Design review of the part built by this model. Coordinates are the model's own, in mm. A direction names the side the tool comes from. Coordinates: 2 decimals unless noted, no trailing zeros. Write each loop counter-clockwise with the first axis right and the second up, starting at its lowest first coordinate (ties: lowest second). Pieces come first, ordered by that corner, then holes.
Q1. Machinability: for faces 1 (the flat face through (-3.75, 3, 40)), 2 (the cylindrical face through (-32.93, 2.03, 49.4)), 3 (the flat face through (4, 2.5, -3)), 4 (the flat face through (-26, 2, -27)), 5 (the flat face through (20.5, 3, 16)), which of the approach directions +Z, -Z, +X, -X, +Y, -Y give a long, thin tool a straight path to every point of the face, cutting with its end or side? Answer none if there is none.
Q2. Take a section at C-C (x = 16). State how many separate pieces and enclosed holes the cut face has, and give its area (3 significant figures).
Q3. Mouldability with a two-part tool opening along X and no side actions: class faces 6 (the flat face through (29, 3, 35.5)), 7 (the cylindrical face through (32.93, 2.03, -49.4)), 8 (the flat face through (5, 1, -3.5)) as pulls with the +X half, pulls with the -X half, needs draft (parallel to the pull), parting line crosses it, or undercut.
Q4. Take a section at A-A (z = -13). Give the boundary of the cut face in (x, y), and give its area (3 significant figures).
Q5. For probe 1 along Z at (x, y) = (-31, 3.55); probe 2 along X at (y, z) = (0.2, -32); probe 3 along X at (y, z) = (2.2, -6), list the stretches that pass through material, from the lowest coordinate up.
Q6. Take a section at B-B (x = 26). Give the boundary of the cut face in (y, z), and give its area (3 significant figures).
Q7. Insertion check: pin 1 (1 mm diameter, centred on x = -23.5, y = 3, fed in from +Z); pin 2 (0.8 mm diameter, centred on x = -25.5, z = -28, fed in from -Y); pin 3 (3.5 mm diameter, centred on x = -27.5, z = -28.5, fed in from -Y). Each pin has a flat end and moves straight along its axis. Give the tip position at first contact, or say it passes through.
Autodesk Inventor part; units mm, degrees
ref_plane "YZ Plane" through (0, 0, 0) normal (1, 0, 0) x (0, 1, 0)
ref_plane "XZ Plane" through (0, 0, 0) normal (0, 1, 0) x (-1, 0, 0)
ref_plane "XY Plane" through (0, 0, 0) normal (0, 0, 1) x (1, 0, 0)
sketch "Sketch2" plane through (0, 0, 0) normal (0, 1, 0) x (-1, 0, 0)
  line L0 (-33.5, -50) -> (33.5, -50)
  line L1 (33.5, -50) -> (33.5, 50)
  line L2 (33.5, 50) -> (-33.5, 50)
  line L3 (-33.5, 50) -> (-33.5, -50)
  line L4 (-33.5, -50) -> (33.5, 50) construction
  line L5 (33.5, -50) -> (-33.5, 50) construction
  point P0 (0, 0)
  dimension "d0" = 67
  dimension "d1" = 100
extrude "Extrusion1" add sketch "Sketch2" along normal blind 4
sketch "Sketch3" plane through (0, 4, 0) normal (0, 1, 0) x (1, 0, 0)
  line L0 (33.5, 50) -> (-33.5, 50)
  line L1 (-14.5, -6.5) -> (23.5, -6.5)
  line L2 (23.5, -6.5) -> (23.5, 46)
  line L3 (23.5, 46) -> (-14.5, 46)
  line L4 (-14.5, 46) -> (-14.5, -6.5)
  line L5 (-14.5, -6.5) -> (23.5, 46) construction
  line L6 (23.5, -6.5) -> (-14.5, 46) construction
  line L7 (33.5, -50) -> (33.5, 50)
  point P0 (0, 0)
  point P1 (4.5, 19.75)
  dimension "d4" = 38
  dimension "d5" = 52.5
  dimension "d6" = 4
  dimension "d99" = 10
extrude "Extrusion2" cut sketch "Sketch3" against normal blind 1.5
sketch "Sketch4" plane through (0, 2.5, 0) normal (0, 1, 0) x (1, 0, 0)
  line L0 (23.5, -6.5) -> (-14.5, -6.5)
  line L1 (23.5, 46) -> (23.5, -6.5)
  line L2 (-14.5, 46) -> (23.5, 46)
  line L3 (-14.5, -6.5) -> (-14.5, 46)
  line L4 (-12, 44.5) -> (21, 44.5)
  line L5 (21, 44.5) -> (21, 3.5)
  line L6 (21, 3.5) -> (-12, 3.5)
  line L7 (-12, 3.5) -> (-12, 44.5)
  line L8 (-12, 44.5) -> (21, 3.5) construction
  line L9 (21, 44.5) -> (-12, 3.5) construction
  point P0 (0, 0)
  point P1 (4.5, 24)
  dimension "d9" = 10
  dimension "d10" = 1.5
  dimension "d11" = 2.5
  dimension "d12" = 2.5
extrude "Extrusion3" cut sketch "Sketch4" against normal blind 2.5 contours L4 L5 L6 L7
sketch "Sketch5" plane through (0, 4, 0) normal (0, 1, 0) x (1, 0, 0)
  line L0 (23.5, 46) -> (23.5, -6.5)
  line L1 (23.5, -6.5) -> (-14.5, -6.5)
  line L2 (-14.5, -6.5) -> (-14.5, 46)
  line L3 (-12.5, -13) -> (-12.5, -6.5)
  line L4 (21.5, -13) -> (21.5, -6.5)
  line L5 (33.5, 50) -> (-33.5, 50)
  line L6 (-12.5, -13) -> (21.5, -13)
  point P0 (0, 0)
  dimension "d18" = 2
  dimension "d19" = 2
  dimension "d158" = 6.5
extrude "Extrusion4" cut sketch "Sketch5" against normal blind 0.25
sketch "Sketch12" plane through (0, 4, 0) normal (0, 1, 0) x (1, 0, 0)
  line L0 (21.5, -13) -> (-12.5, -13)
  line L1 (-13.5, -37) -> (24.5, -37)
  line L2 (24.5, -37) -> (24.5, -13)
  line L3 (24.5, -13) -> (-13.5, -13)
  line L4 (-13.5, -13) -> (-13.5, -37)
  line L5 (-13.5, -37) -> (24.5, -13) construction
  line L6 (24.5, -37) -> (-13.5, -13) construction
  line L7 (23.5, 46) -> (23.5, -6.5)
  point P0 (0, 0)
  point P1 (5.5, -25)
  point P2 (5.5, -25)
  dimension "d58" = 38
  dimension "d59" = 24
  dimension "d100" = 1
extrude "Extrusion10" cut sketch "Sketch12" against normal blind 4
sketch "Sketch13" plane through (24.5, 4, 13) normal (-1, 0, 0) x (0, 0, 1)
  line L0 (0, 0) -> (24, 0)
  line L1 (0, 0) -> (0, -4)
  line L2 (24, -4) -> (0, -4)
  line L3 (6, 0) -> (6, -4)
  line L4 (0, -2.2) -> (6, -2.2)
  point P0 (-13, -4)
  dimension "d67" = 6
  dimension "d74" = 1.8
sketch "Sketch14" plane through (-13.5, 4, 37) normal (1, 0, 0) x (0, 0, -1)
  line L0 (0, 0) -> (24, 0)
  line L1 (0, 0) -> (0, -4)
  line L2 (4, -2.2) -> (4, 0)
  line L3 (24, -4) -> (0, -4)
  line L4 (0, -2.2) -> (4, -2.2)
  point P0 (37, -4)
  point P1 (0, -2)
  dimension "d79" = 1.8
  dimension "d180" = 4
extrude "Extrusion13" add sketch "Sketch13" along normal blind 4 contours L0 L3 L4 L1
extrude "Extrusion14" add sketch "Sketch14" along normal blind 6
sketch "Sketch16" plane through (0, 3.75, 0) normal (0, 1, 0) x (1, 0, 0)
  line L0 (-12.5, -13) -> (-12.5, -6.5)
  line L1 (20.5, -13) -> (-12.5, -13)
  line L2 (21.5, -13) -> (20.5, -13)
  line L3 (21.5, -6.5) -> (21.5, -13)
  line L4 (-12.5, -6.5) -> (21.5, -6.5)
  point P0 (0, 0)
extrude "Extrusion15" cut sketch "Sketch16" against normal up to next
sketch "Sketch17" plane through (21.5, 4, 6.5) normal (-1, 0, 0) x (0, 0, 1)
  line L0 (0, -1.5) -> (0, -4)
  line L1 (6.5, -4) -> (0, -4)
  line L2 (6.5, 0) -> (6.5, -2.2)
  line L3 (0, -1.5) -> (-1.7339, -1.5) construction
  spline S0 degree 4 poles (0, -1.5) (0.1402, -1.5095) (0.2435, -1.6356) (0.3737, -1.9813) (0.553, -2.595) (1.1197, -3.1548) (2.0475, -3.4989) (2.9931, -3.3708) (3.499, -3.5451) (3.8409, -4) knots 0 0 0 0 0 0.170303 0.299552 0.400825 0.520493 0.699331 1 1 1 1 1
  line L4 (3.4081, -3.4241) -> (4.2737, -4.5759) construction
  arc A0 (4.1216, -4.4884) -> (3.4499, -3.5946) centre (2.0035, -5.3809) ccw construction
  line L5 (0.8397, -2.9601) -> (1.8217, -3.4241) construction
  arc A1 (0.9695, -2.9668) -> (1.7341, -3.3281) centre (2.1148, -1.5326) ccw construction
  line L6 (-0.6498, -1.456) -> (0.6498, -1.544) construction
  arc A2 (0.2995, -1.6769) -> (-0.3206, -1.6349) centre (-0.0262, -1.8863) ccw construction
  line L7 (0.2788, -1.8046) -> (0.6778, -2.7982) construction
  point P0 (-6.5, -4)
  point P1 (0.2332, -1.6655)
  point P2 (0.4783, -2.3014)
  point P3 (1.3307, -3.1921)
  point P4 (2.6959, -3.4298)
  point P5 (2.8138, -1.3633)
  point P6 (0.354, -1.8963)
  point P7 (0.6678, -2.6804)
extrude "Extrusion16" add sketch "Sketch17" along normal up to next
sketch "Sketch18" plane through (0, 4, 0) normal (0, 1, 0) x (1, 0, 0)
  line L0 (-33.5, 50) -> (-33.5, -50)
  line L1 (-32.5, 44) -> (-19.5, 44)
  line L2 (-19.5, 44) -> (-19.5, 12)
  line L3 (-19.5, 12) -> (-32.5, 12)
  line L4 (-32.5, 12) -> (-32.5, 44)
  line L5 (33.5, 50) -> (-33.5, 50)
  point P0 (0, 0)
  dimension "d89" = 1
  dimension "d97" = 13
  dimension "d98" = 32
  dimension "d157" = 6
extrude "Extrusion17" cut sketch "Sketch18" against normal up to next
sketch "Sketch19" plane through (-32.5, 4, -12) normal (1, 0, 0) x (0, 0, -1)
  line L0 (0, 0) -> (0, -4)
  line L1 (14.5, -2) -> (17.5, -2)
  line L2 (17.5, -2) -> (17.5, 0)
  line L3 (17.5, 0) -> (14.5, 0)
  line L4 (14.5, 0) -> (14.5, -2)
  line L5 (14.5, -2) -> (17.5, 0) construction
  line L6 (17.5, -2) -> (14.5, 0) construction
  line L7 (0, 0) -> (32, 0)
  point P0 (16, -1)
  dimension "d106" = 3
  dimension "d107" = 2
  dimension "d108" = 16
extrude "Extrusion18" add sketch "Sketch19" along normal up to next
sketch "Sketch21" plane through (-32.5, 2, -29.5) normal (0, -1, 0) x (1, 0, 0)
  line L0 (5, 0) -> (8, 0)
  line L1 (8, 0) -> (8, 2)
  line L2 (8, 2) -> (5, 2)
  line L3 (5, 2) -> (5, 0)
  line L4 (5, 0) -> (8, 2) construction
  line L5 (8, 0) -> (5, 2) construction
  line L6 (0, 0) -> (13, 0)
  point P0 (-32.5, -3.5)
  point P1 (6.5, 1)
  point P2 (6.5, 1)
  point P3 (6.5, 1)
  point P4 (6.5, 0)
  dimension "d111" = 3
  dimension "d112" = 2
extrude "Extrusion19" cut sketch "Sketch21" against normal blind 0.5
fillet "Fillet6" radius 1 1 edges at (-26, 2.5, -29.5)
sketch "Sketch22" plane through (-32.5, 2, -29.5) normal (0, -1, 0) x (1, 0, 0)
  line L0 (13, 0) -> (13, 3)
  circle A0 centre (2.375, 1.5) radius 1.25
  circle A1 centre (10.625, 1.5) radius 1.25
  line L1 (0, 3) -> (13, 3)
  line L2 (0, 0) -> (0, 3)
  line L3 (0, 0) -> (5, 0)
  point P0 (6.5, 1.5)
  point P1 (6.5, 3)
  point P2 (13, 1.5)
  point P3 (0, 1.5)
  point P4 (6.5, 3)
  dimension "d116" = 2.5
  dimension "d117" = 2.5
  dimension "d118" = 8.25
  dimension "d119" = 4.125
extrude "Extrusion20" add sketch "Sketch22" along normal blind 2
chamfer "Chamfer3" distance 0.5 angle 45 2 edges at (-31.375, 0, -28) (-23.125, 0, -28)
sketch "Sketch23" plane through (0, 4, 0) normal (0, 1, 0) x (1, 0, 0)
  line L0 (-33.5, 50) -> (-33.5, -50)
  line L1 (-33.5, -50) -> (33.5, -50)
  line L2 (-25.75, -34) -> (-15.25, -34)
  line L3 (-15.25, -34) -> (-15.25, -50)
  line L4 (-15.25, -50) -> (-25.75, -50)
  line L5 (-25.75, -50) -> (-25.75, -34)
  line L6 (-25.75, -34) -> (-15.25, -50) construction
  line L7 (-15.25, -34) -> (-25.75, -50) construction
  line L8 (21.5, -6.5) -> (21.5, -13)
  line L9 (-25.5, -34) -> (-25.5, -42)
  line L10 (-25.5, -42) -> (-25.75, -42)
  line L11 (-15.5, -34) -> (-15.5, -42)
  line L12 (-15.5, -42) -> (-15.25, -42)
  point P0 (0, 0)
  point P1 (-20.5, -42)
  dimension "d125" = 10.5
  dimension "d126" = 16
  dimension "d127" = 13
  dimension "d130" = 0.25
  dimension "d131" = 0.25
  dimension "d132" = 8
extrude "Extrusion22" cut sketch "Sketch23" against normal blind 2.5 contours L5 L10 L9 L2 L11 L12 L3 L1
sketch "Sketch25" plane through (0, 4, 0) normal (0, 1, 0) x (1, 0, 0)
  line L0 (33.5, -50) -> (33.5, 50)
  line L1 (24.5, -19) -> (24.5, -37)
  line L2 (24.5, -37) -> (-7.5, -37)
  line L3 (24.5, -19) -> (33.5, -19)
  line L4 (24.5, -35.5) -> (33.5, -35.5)
  point P0 (0, 0)
  dimension "d150" = 1.5
extrude "Extrusion24" cut sketch "Sketch25" against normal blind 2
sketch "Sketch27" plane through (0, 4, 0) normal (0, 1, 0) x (1, 0, 0)
  line L0 (-15.25, -50) -> (33.5, -50)
  line L1 (24.5, -35.5) -> (24.5, -37)
  line L2 (-4, -42) -> (8.5, -42)
  line L3 (8.5, -42) -> (8.5, -50)
  line L4 (8.5, -50) -> (-4, -50)
  line L5 (-4, -50) -> (-4, -42)
  line L6 (-4, -42) -> (8.5, -50) construction
  line L7 (8.5, -42) -> (-4, -50) construction
  line L8 (-3.75, -37) -> (8.25, -37)
  line L9 (8.25, -37) -> (8.25, -42)
  line L10 (8.25, -42) -> (-3.75, -42)
  line L11 (-3.75, -42) -> (-3.75, -37)
  line L12 (-3.75, -37) -> (8.25, -42) construction
  line L13 (8.25, -37) -> (-3.75, -42) construction
  line L14 (24.5, -37) -> (-7.5, -37)
  point P0 (0, 0)
  point P1 (2.25, -46)
  point P2 (2.25, -39.5)
  point P3 (2.25, -39.5)
  point P4 (2.25, -46)
  dimension "d166" = 12.5
  dimension "d167" = 8
  dimension "d168" = 12
  dimension "d170" = 16
extrude "Extrusion26" cut sketch "Sketch27" against normal blind 2.5
sketch "Sketch29" plane through (0, 1.5, 0) normal (0, 1, 0) x (1, 0, 0)
  line L0 (-3.75, -37) -> (8.25, -37)
  line L1 (-3.75, -42) -> (-3.75, -37)
  line L2 (8.25, -37) -> (8.25, -42)
  line L3 (-3.75, -38) -> (8.25, -38)
  point P0 (0, 0)
  dimension "d177" = 1
extrude "Extrusion28" add sketch "Sketch29" along normal blind 0.5
sketch "Sketch30" plane through (0, 4, 0) normal (0, 1, 0) x (1, 0, 0)
  line L0 (-27.25, 12) -> (-27.25, -26.8211)
  line L1 (-27.25, -26.8211) -> (-23, -31.0711)
  line L2 (-23, -31.0711) -> (-23, -34)
  line L3 (-24.75, 12) -> (-24.75, -22.25)
  line L4 (-24.75, -22.25) -> (-18, -29)
  line L5 (-18, -29) -> (-18, -34)
  line L6 (-25.5, -34) -> (-15.5, -34)
  line L7 (-32.5, 12) -> (-19.5, 12)
  line L8 (-27.25, 12) -> (-24.75, 12)
  line L9 (-23, -34) -> (-18, -34)
  line L10 (-25.5, -34) -> (-15.5, -34)
  point P0 (0, 0)
  point P1 (-20.5, -34)
  point P2 (-20.5, -34)
  point P3 (-26, 12)
  point P4 (-26, 12)
  point P5 (-20.5, -34)
  point P6 (-26, 12)
  dimension "d181" = 2.5
  dimension "d182" = 5
  dimension "d183" = 45
  dimension "d184" = 45
  dimension "d185" = 2.5
  dimension "d186" = 1.25
  dimension "d188" = 5
  dimension "d189" = 5
extrude "Extrusion29" cut sketch "Sketch30" against normal blind 2.5
chamfer "Chamfer5" distance 2 angle 45 2 edges at (-27.25, 2.75, -12) (-24.75, 2.75, -12)
fillet "Fillet9" radius 2 10 edges at (-23, 2.75, 34) (-18, 2.75, 34) (-18, 2.75, 29) (-24.75, 2.75, 22.25) (-24.75, 2.75, -10) (-22.75, 2.75, -12) (-29.25, 2.75, -12) (-27.25, 2.75, -10) (-27.25, 2.75, 26.8211) (-23, 2.75, 31.0711)
fillet "Fillet10" radius 2 4 edges at (33.5, 2, 50) (-33.5, 2, 50) (33.5, 2, -50) (-33.5, 2, -50)
properties part number "DisplayTop"
Response:
1. face 1: +Z, +Y
1. face 2: +Z, -X, +Y, -Y
1. face 3: +Y
1. face 4: -Y
1. face 5: +Y, -Y
2. separate pieces: 3
2. enclosed holes: 0
2. area: 100 mm2
3. face 6: needs draft
3. face 7: pulls with the +X half
3. face 8: undercut
4. outline: (-33.5, 0) - (-32.5, 0) - (-32.5, 4) - (-33.5, 4) - close; (-19.5, 0) - (-12, 0) - (-12, 2.5) - (-14.5, 2.5) - (-14.5, 4) - (-19.5, 4) - close; (21, 0) - (33.5, 0) - (33.5, 4) - (23.5, 4) - (23.5, 2.5) - (21, 2.5) - close
4. area: 76.5 mm2
5. probe 1: z = -50 to -44, -29.5 to -26.5, -12 to 50
5. probe 2: x = -33.5 to -32.5, -19.5 to -12, 21 to 33.5
5. probe 3: x = -33.5 to -27.25, -24.75 to -12, 21 to 33.5
6. outline: (0, -50) - (4, -50) - (4, 19) - (2, 19) - (2, 35.5) - (4, 35.5) - (4, 50) - (0, 50) - close
6. area: 367 mm2
7. pin 1: stops at z = 33.73
7. pin 2: stops at y = 2.5
7. pin 3: stops at y = 0.17
